```python
from build123d import *

# Parameters (mm, degrees)
SKETCH_1_W          = 15
SKETCH_1_H          = 15
SKETCH_1_W_2        = 13
SKETCH_1_H_2        = 13
EXTRUDE_1_DEPTH     = 250
SKETCH_2_R          = 1.5
CUT_EXTRUDE_1_DEPTH = 250
SKETCH_3_R          = 4
CUT_EXTRUDE_2_DEPTH = 10
SKETCH_4_R          = 4
CUT_EXTRUDE_3_DEPTH = 10


with BuildPart() as part:
    # 草图1 → 凸台-拉伸1 (new body)
    with BuildSketch(Plane(origin=(0, 0, 0), x_dir=(0, 0, -1), z_dir=(1, 0, 0))):
        Rectangle(SKETCH_1_W, SKETCH_1_H)
        Rectangle(SKETCH_1_W_2, SKETCH_1_H_2, mode=Mode.SUBTRACT)
    extrude(amount=EXTRUDE_1_DEPTH)

    # 草图2 → 切除-拉伸1 (cut)
    with BuildSketch(Plane(origin=(0, 7.5, 0), x_dir=(1, 0, 0), z_dir=(0, 1, 0))):
        with Locations(Location((30, 0, 0), (0, 0, 270))):
            Circle(SKETCH_2_R)
        with Locations(Location((60, 0, 0), (0, 0, 270))):
            Circle(SKETCH_2_R)
        with Locations(Location((190, 0, 0), (0, 0, 90))):
            Circle(SKETCH_2_R)
        with Locations(Location((220, 0, 0), (0, 0, 90))):
            Circle(SKETCH_2_R)
    extrude(amount=-CUT_EXTRUDE_1_DEPTH, mode=Mode.SUBTRACT)

    # 草图3 → 切除-拉伸2 (cut)
    with BuildSketch(Plane(origin=(0, 7.5, 0), x_dir=(1, 0, 0), z_dir=(0, 1, 0))):
        with Locations(Location((30, 0, 0), (0, 0, 270))):
            Circle(SKETCH_3_R)
        with Locations(Location((220, 0, 0), (0, 0, 270))):
            Circle(SKETCH_3_R)
    extrude(amount=-CUT_EXTRUDE_2_DEPTH, mode=Mode.SUBTRACT)

    # 草图4 → 切除-拉伸3 (cut)
    with BuildSketch(Plane.XZ.offset(7.5)):
        with Locations(Location((60, 0, 0), (0, 0, 270))):
            Circle(SKETCH_4_R)
        with Locations(Location((190, 0, 0), (0, 0, 270))):
            Circle(SKETCH_4_R)
    extrude(amount=-CUT_EXTRUDE_3_DEPTH, mode=Mode.SUBTRACT)


solid = part.part
```
Geometry: final body of the model. Coordinates: model frame, mm. A direction names the side the tool comes from. Coordinates: 2 decimals unless noted, no trailing zeros. Loops run counter-clockwise (first coordinate to the right, second up) from the corner with the lowest first, then second, coordinate; pieces in that order, holes last. Notation, with made-up numbers: M -15.75,-33 L -9.75,-33 A29 cw -9.75,2 Z; hole C -27,71 d7. An arc over 180 degrees is marked long. Put each result on its own line as item: value.
(1) Cut plane A-A on x = 206. Return the cut outline in (y, z).
Answer sheet:
outline: M -7.5,-7.5 L 7.5,-7.5 L 7.5,7.5 L -7.5,7.5 Z; hole M -6.5,-6.5 L 6.5,-6.5 L 6.5,6.5 L -6.5,6.5 Z
(2) Draft query along X for faces 6 (the face through (250, 0, 7)), 7 (the face through (123, 0, -7.5)), 8 (the face through (0, 0, 7)), 9 (the face through (223.373, 7.007, 2.15)). Return one class per face: pulls with the +X half, pulls with the -X half, needs draft (parallel to the pull), parting line crosses it, or undercut.
Answer sheet:
face 6: pulls with the +X half
face 7: needs draft
face 8: pulls with the -X half
face 9: undercut
(3) Access query for faces 1 (the face through (123, -7.5, 0)), 2 (the face through (56.095, -7.007, 0.867)), 3 (the face through (123, 7.5, 0)), 4 (the face through (33.966, 7.007, -0.521)), 5 (the face through (123, -6.5, 0)). Directions: +Z, -Z, +X, -X, +Y, -Y. A direction counts if a zero-diameter tool reaches every point of the face in a straight line with its end or side. Return the directions, or none.
Answer sheet:
face 1: +Z, -Z, +X, -X, -Y
face 2: -Y
face 3: +Z, -Z, +X, -X, +Y
face 4: +Y
face 5: +X, -X
(4) First-contact query: pin 1 (1.8 mm diameter, centred on x = 60, z = 0, fed in from -Y). Flat tip, straight axial feed; report the tip coordinate or a pass-through.
Answer sheet:
pin 1: passes through
(5) Cut plane B-B on y = 0.25. Return the cut outline in (x, z).
Answer sheet:
outline: M 0,-7.5 L 250,-7.5 L 250,-6.5 L 0,-6.5 Z; M 0,6.5 L 250,6.5 L 250,7.5 L 0,7.5 Z
(6) Material intervals for probe 1 along X at (y, z) = (6.8, 0); probe 2 along X at (y, z) = (-7.3, 0); probe 3 along Y at (x, z) = (121, -5.25), sorted ascending.
Answer sheet:
probe 1: x = 0 to 26, 34 to 58.5, 61.5 to 188.5, 191.5 to 216, 224 to 250
probe 2: x = 0 to 28.5, 31.5 to 56, 64 to 186, 194 to 218.5, 221.5 to 250
probe 3: y = -7.5 to -6.5, 6.5 to 7.5
